Design review of the part shown in the three views and the two pictorial views. Dimensions are in mm from the part's minimum x, y and z. Give positions to 0.01 mm unless a question says otherwise; leave off trailing zeros. Loops run counter-clockwise (first coordinate to the right, second up) from the corner with the lowest first, then second, coordinate; pieces in that order, holes last. Notation, with made-up numbers: M 85.25,-2 L 91.25,-2 A15 cw 91.25,22 Z; hole C -31,20.25 d7. An arc over 180 degrees is marked long. Return JSON: item names as keys, results as strings. Group by question number.
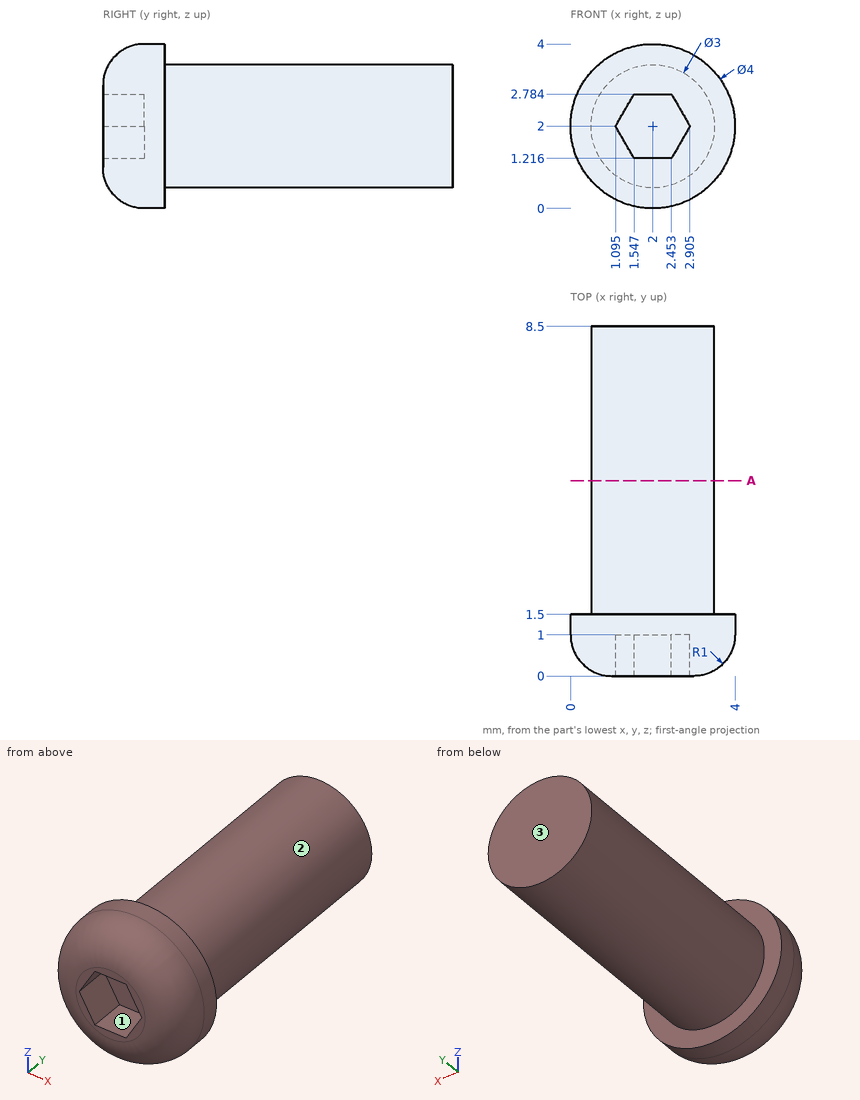
(1) For pin 1 (0.5 mm diameter, centred on x = 2, z = 2, fed in from -Y); pin 2 (1.5 mm diameter, centred on x = 2, y = 6, fed in from -Z); pin 3 (2 mm diameter, centred on x = 3.5, z = 1.5, fed in from +Y); pin 4 (2 mm diameter, centred on x = 1.5, y = 3, fed in from +Z), all flat-tipped, find the tip position at first contact; note any pin that passes through.
(2) Mouldability with a two-part tool opening along X and no side actions: class the marked faces 1, 2 and 3 as released by +X, released by -X, zero draft, split by the parting line, or undercut.
(3) Add section A-A (y = 4.75). Write out the cut boundary in (x, z).
(4) For probe 1 along X at (y, z) = (2.5, 2); probe 2 along Y at (x, z) = (2.35, 2.25); probe 3 along Y at (x, z) = (3.3, 1), list the stretches that pass through material, from the lowest coordinate up.
Verdict:
{
 "1": {"pin 1": "stops at y = 1", "pin 2": "stops at z = 0.5", "pin 3": "stops at y = 8.5", "pin 4": "stops at z = 3.5"},
 "2": {"face 1": "undercut", "face 2": "split by the parting line", "face 3": "zero draft"},
 "3": {"outline": "C 2,2 d3"},
 "4": {"probe 1": "x = 0.5 to 3.5", "probe 2": "y = 1 to 8.5", "probe 3": "y = 0.23 to 1.5"}
}
